Print and shaded views of the part. All mm, measured from the part's lowest x, y and z. A direction names the side the tool comes from. Round coordinates to 2 decimals unless told otherwise and drop trailing zeros. Order: outer loops, then holes, each group sorted by start corner. A loop starts at its lowest first (then second) coordinate and runs counter-clockwise, first axis right, second up. Notation, with made-up numbers: (-20.75, -21.75) - (5.25, -21.75) arc R19 ccw to (5.25, 13.25) - close; hole circle Ø11 at (77.25, 4). An arc over 180 degrees is marked (long way). Return JSON: item names as keys, results as strings. Group by question number.
Item 1: Probe probe 1 along X at (y, z) = (13, 20); probe 2 along Y at (x, z) = (27, 35.5); probe 3 along Z at (x, y) = (21, 7.5). List the from-to ranges inside material, lowest first.
Item 2: Saw through at D-D on z = 5. List the corners of the cut face in (x, y).
Item 3: Saw through at A-A on y = 5.75. List the corners of the cut face in (x, z).
Item 4: Two-plate mould, pull along Z, no slides. Class the marked faces 1, 2 and 3: released by +Z, released by -Z, zero draft, split by the parting line, or undercut.
Item 5: Saw through at B-B on z = 13.5. List the corners of the cut face in (x, y), and give its area (3 significant figures).
Item 6: Drop flat-ended pins along their axis: pin 1 (8 mm diameter, centred on y = 9, z = 26, fed in from -X); pin 2 (4 mm diameter, centred on x = 26.5, y = 11.5, fed in from -Z); pin 3 (1 mm diameter, centred on x = 22, z = 34.5, fed in from -Y); pin 4 (1 mm diameter, centred on y = 11.5, z = 22, fed in from +X). Give the stop position or say it passes through.
Item 7: Saw through at C-C on x = 37.5. List the corners of the cut face in (y, z), and give its area (3 significant figures).
Item 8: Tool access for the marked faces 4 and 5: list every direction of +Z, -Z, +X, -X, +Y, -Y with a clear straight run to the whole face (end or side of a thin tool).
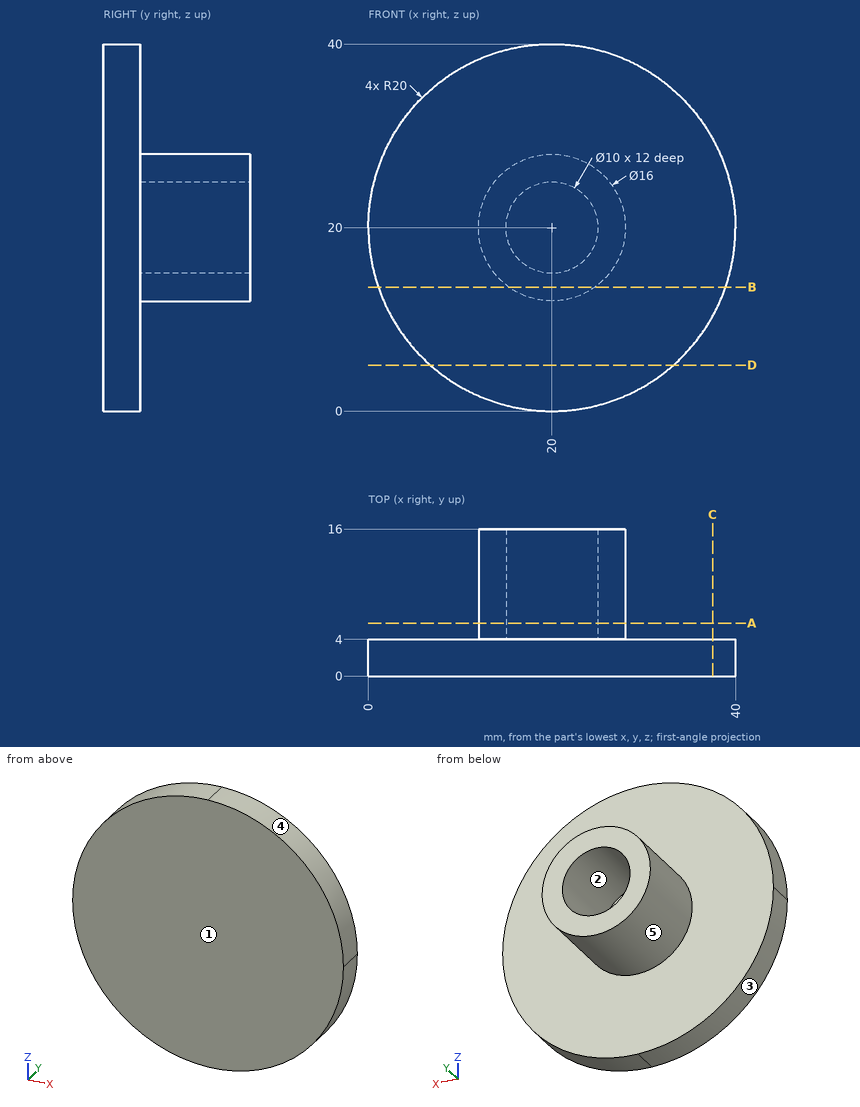
Filled in:
{
 "1": {"probe 1": "x = 12 to 15, 25 to 28", "probe 2": "y = 0 to 4", "probe 3": "z = 12.06 to 15.1, 24.9 to 27.94"},
 "2": {"outline": "(6.77, 0) - (33.23, 0) - (33.23, 4) - (6.77, 4) - close"},
 "3": {"outline": "circle Ø16 at (20, 20); hole circle Ø10 at (20, 20)"},
 "4": {"face 1": "zero draft", "face 2": "undercut", "face 3": "released by -Z"},
 "5": {"outline": "(1.09, 0) - (38.91, 0) - (38.91, 4) - (24.66, 4) - (24.66, 16) - (15.34, 16) - (15.34, 4) - (1.09, 4) - close", "area": "263 mm^2"},
 "6": {"pin 1": "stops at x = 12.25", "pin 2": "stops at z = 13.39", "pin 3": "stops at y = 0", "pin 4": "stops at x = 27.86"},
 "7": {"outline": "(0, 10.32) - (4, 10.32) - (4, 29.68) - (0, 29.68) - close", "area": "77.5 mm^2"},
 "8": {"face 4": "+Z, +X, +Y, -Y", "face 5": "+Y"}
}
